Work out the finished part from the listing and answer in its coordinate system (mm). Coordinates: 2 decimals unless noted, no trailing zeros. Order: outer loops, then holes, each group sorted by start corner. A loop starts at its lowest first (then second) coordinate and runs counter-clockwise, first axis right, second up. Notation, with made-up numbers: M 53,36.5 L 106,36.5 A29 cw 106,66.5 Z; hole C 27.25,17 d6. An arc over 180 degrees is marked long. Answer in a Markdown table with one row per item. Add a question column.
Item 1: The part is cut by section B-B (z = 337.5). Write down the section's boundary in (x, y).
Item 2: Consider line 1 (X direction, y = 3.5, z = 356.5); line 2 (Y direction, x = -6.75, z = 119); line 3 (X direction, y = 6.25, z = 304). Determine where each line is inside the solid, lowest interval first. Write a range as from..to.
Item 3: Flat-ended cylindrical pins translate along their axes: pin 1 Ø3.5 at (x, z) = (0, 10) entering from +Y; pin 2 Ø8 at (x, z) = (0, 356.5) entering from +Y; pin 3 Ø1.9 at (y, z) = (10, 246) entering from +X. Find the tip coordinate at first contact, or state that the pin passes through.
Item 4: The part is cut by section A-A (y = 2). State how many separate pieces and enclosed holes the cut face has, then the cut area to 3 significant figures.
from build123d import *

# Parameters (mm, degrees)
SALIENTE_EXTRUIR1_DEPTH = 655
CROQUIS2_R              = 3
CORTAR_EXTRUIR1_DEPTH   = 12


with BuildPart() as part:
    # Croquis1 → Saliente-Extruir1 (new body)
    with BuildSketch(Plane.XY):
        with BuildLine():
            Line((-10, 0), (-10, 5.656056356))
            ThreePointArc((-10, 5.656056356), (-8.921539569, 7.959897862), (-6.461542876, 8.607338099))
            Line((-6.461542876, 8.607338099), (-5.221744043, 9.236902282))
            Line((-5.221744043, 9.236902282), (-7.354818693, 9.236902282))
            Line((-7.354818693, 9.236902282), (-7.354818693, 11))
            Line((-7.354818693, 11), (7.354818693, 11))
            Line((7.354818693, 11), (7.354818693, 9.236902282))
            Line((7.354818693, 9.236902282), (5.221744043, 9.236902282))
            Line((5.221744043, 9.236902282), (6.461542876, 8.607338099))
            ThreePointArc((6.461542876, 8.607338099), (8.921539569, 7.959897862), (10, 5.656056356))
            Line((10, 5.656056356), (10, 0))
            Line((10, 0), (0, 0))
            Line((0, 0), (-10, 0))
        make_face()
    extrude(amount=SALIENTE_EXTRUIR1_DEPTH)

    # Croquis2 → Cortar-Extruir1 (cut)
    with BuildSketch(Plane(origin=(0, 11, 0), x_dir=(1, 0, 0), z_dir=(0, 1, 0))):
        with Locations((0, -10)):
            Circle(CROQUIS2_R)
        with Locations((0, -48.5)):
            Circle(CROQUIS2_R)
        with Locations((0, -87)):
            Circle(CROQUIS2_R)
        with Locations((0, -125.5)):
            Circle(CROQUIS2_R)
        with Locations((0, -164)):
            Circle(CROQUIS2_R)
        with Locations((0, -202.5)):
            Circle(CROQUIS2_R)
        with Locations((0, -241)):
            Circle(CROQUIS2_R)
        with Locations((0, -279.5)):
            Circle(CROQUIS2_R)
        with Locations((0, -318)):
            Circle(CROQUIS2_R)
        with Locations((0, -356.5)):
            Circle(CROQUIS2_R)
        with Locations((0, -395)):
            Circle(CROQUIS2_R)
        with Locations((0, -433.5)):
            Circle(CROQUIS2_R)
        with Locations((0, -472)):
            Circle(CROQUIS2_R)
        with Locations((0, -510.5)):
            Circle(CROQUIS2_R)
        with Locations((0, -549)):
            Circle(CROQUIS2_R)
        with Locations((0, -587.5)):
            Circle(CROQUIS2_R)
        with Locations((0, -626)):
            Circle(CROQUIS2_R)
    extrude(amount=-CORTAR_EXTRUIR1_DEPTH, mode=Mode.SUBTRACT)


solid = part.part
Reply:
| question | item | result |
|---|---|---|
| 1 | outline | M -10,0 L 10,0 L 10,5.66 A3 ccw 6.46,8.61 L 5.22,9.24 L 7.35,9.24 L 7.35,11 L -7.35,11 L -7.35,9.24 L -5.22,9.24 L -6.46,8.61 A3 ccw -10,5.66 Z |
| 2 | line 1 | x = -10..-3, 3..10 |
| 2 | line 2 | y = 0..8.65, 9.24..11 |
| 2 | line 3 | x = -9.94..9.94 |
| 3 | pin 1 | passes through |
| 3 | pin 2 | stops at y = 11 |
| 3 | pin 3 | stops at x = 7.35 |
| 4 | separate pieces | 1 |
| 4 | enclosed holes | 17 |
| 4 | area | 12,600 mm2 |
